from build123d import *

# Parameters (mm, degrees)
SKETCH1_R           = 12.5
BOSS_EXTRUDE2_DEPTH = 12
CUT_EXTRUDE3_REACH  = 14
SKETCH5_R           = 2.125
BOSS_EXTRUDE3_DEPTH = 12
SKETCH9_W           = 8
SKETCH9_H           = 10
CUT_EXTRUDE4_DEPTH  = 10
SKETCH10_W          = 8
SKETCH10_H          = 10
CUT_EXTRUDE5_DEPTH  = 10
SKETCH11_R          = 2
CUT_EXTRUDE6_DEPTH  = 21.229774891
SKETCH12_R          = 2
CUT_EXTRUDE7_DEPTH  = 30.012682497


with BuildPart() as part:
    # Sketch1 → Boss-Extrude2 (new body)
    with BuildSketch(Plane.XY):
        Circle(SKETCH1_R)
    extrude(amount=BOSS_EXTRUDE2_DEPTH)

    # Sketch5 → Cut-Extrude3 (cut, up to next)
    with BuildSketch(Plane.XY.offset(12), mode=Mode.PRIVATE) as cut_extrude3_sk1:
        Circle(SKETCH5_R)
    cut_extrude3_tool1 = extrude(cut_extrude3_sk1.sketch, amount=-CUT_EXTRUDE3_REACH, mode=Mode.PRIVATE) & part.part
    add(cut_extrude3_tool1.solids().sort_by_distance((0, 0, 12))[0], mode=Mode.SUBTRACT)

    # Sketch6 → Boss-Extrude3 (add)
    with BuildSketch(Plane.XY):
        with BuildLine():
            Line((10.356157589, 7), (20.356157589, 7))
            Line((20.356157589, 7), (20.356157589, -7))
            Line((20.356157589, -7), (10.356157589, -7))
            ThreePointArc((10.356157589, -7), (12.5, 0), (10.356157589, 7))
        make_face()
        with BuildLine():
            Line((-24.231440373, -0.295461436), (-11.458506302, 4.995261088))
            ThreePointArc((-11.458506302, 4.995261088), (-12.259311424, -2.441164357), (-8.670952565, -9.003587153))
            Line((-8.670952565, -9.003587153), (-18.87387232, -13.229774891))
            Line((-18.87387232, -13.229774891), (-20.787289482, -8.610377228))
            Line((-20.787289482, -8.610377228), (-24.231440373, -0.295461436))
        make_face()
    extrude(amount=BOSS_EXTRUDE3_DEPTH)

    # Sketch9 → Cut-Extrude4 (cut)
    with BuildSketch(Plane(origin=(20.356157589, 0, 0), x_dir=(0, 0, -1), z_dir=(1, 0, 0))):
        with Locations((-6, 0)):
            Rectangle(SKETCH9_W, SKETCH9_H)
    extrude(amount=-CUT_EXTRUDE4_DEPTH, mode=Mode.SUBTRACT)

    # Sketch10 → Cut-Extrude5 (cut)
    with BuildSketch(Plane(origin=(-20.787289482, -8.610377228, 0), x_dir=(0, 0, 1), z_dir=(-0.923879533, -0.382683432, 0))):
        with Locations((6, 2)):
            Rectangle(SKETCH10_W, SKETCH10_H)
    extrude(amount=-CUT_EXTRUDE5_DEPTH, mode=Mode.SUBTRACT)

    # Sketch11 → Cut-Extrude6 (cut, through all)
    with BuildSketch(Plane(origin=(0, 7, 0), x_dir=(1, 0, 0), z_dir=(0, 1, 0))):
        with Locations((15.356157589, -6)):
            Circle(SKETCH11_R)
    extrude(amount=-CUT_EXTRUDE6_DEPTH, mode=Mode.SUBTRACT)

    # Sketch12 → Cut-Extrude7 (cut, through all)
    with BuildSketch(Plane(origin=(-3.444150891, 8.314915793, 0), x_dir=(0.923879533, 0.382683432, 0), z_dir=(-0.382683432, 0.923879533, 0))):
        with Locations((-15.587337893, -6)):
            Circle(SKETCH12_R)
    extrude(amount=-CUT_EXTRUDE7_DEPTH, mode=Mode.SUBTRACT)


solid = part.part
Verification items for the finished model (mm, model axes). A direction names the side the tool comes from. Coordinates: 2 decimals unless noted, no trailing zeros. Write each loop counter-clockwise with the first axis right and the second up, starting at its lowest first coordinate (ties: lowest second). Pieces come first, ordered by that corner, then holes. Notation, with made-up numbers: (48.25, 43.5) - (107.25, 43.5) arc R31 cw to (107.25, 76.5) - close; hole circle Ø10 at (-12.75, 44). An arc over 180 degrees is marked (long way). Answer as a JSON object with one key per item and string values.
(1) Gauge pin test, flat ends, axial feed: pin 1 Ø3 at (x, z) = (13.5, 3.5) entering from -Y; pin 2 Ø3 at (x, z) = (14.5, 7.5) entering from +Y; pin 3 Ø2.5 at (x, z) = (15.36, 6) entering from -Y; pin 4 Ø4 at (y, z) = (-8.5, 2.5) entering from -X. Record the tip position at first contact, or that the pin passes through.
Report:
{"pin 1": "y = -7", "pin 2": "y = 7", "pin 3": "through", "pin 4": "x = -21.64"}
(2) Tool access check on faces 1 (the cylindrical face through (-0.958, 12.463, 5.916)), 2 (the flat face through (15, 0, 10)), 3 (the flat face through (-12.34, -2.87, 5.94)). Record the directions out of +Z, -Z, +X, -X, +Y, -Y that give a thin tool (end or side, any length) a straight path to the whole face; none if there is none.
Report:
{"face 1": "+Z, -Z, +Y", "face 2": "+X", "face 3": "none"}
(3) Cross-section at D-D on y = 5.75. Record the cut outline in (x, z), plus the area to 3 significant figures.
Report:
{"outline": "(-11.1, 0) - (20.36, 0) - (20.36, 12) - (-11.1, 12) - close; hole circle Ø4 at (15.36, 6)", "area": "365 mm^2"}
(4) Cross-section at C-C on z = 6. Give the number of separate pieces and of enclosed holes in the cut face, plus the area to 3 significant figures.
Report:
{"separate pieces": "5", "enclosed holes": "1", "area": "517 mm^2"}
(5) Cross-section at B-B on x = 0. Record the cut outline in (y, z) (3 decimals).
Report:
{"outline": "(-12.5, 0) - (-2.125, 0) - (-2.125, 12) - (-12.5, 12) - close; (2.125, 0) - (12.5, 0) - (12.5, 12) - (2.125, 12) - close"}
(6) Thickness scan on line 1 along X through (y, z) = (-0.5, 8.5); line 2 along Y through (x, z) = (10.5, 4.75); line 3 along X through (y, z) = (-1.75, 2.5). Record the ranges inside material, lowest first.
Report:
{"line 1": "-24.15 to -19.5, -13.32 to -2.07, 2.07 to 10.36", "line 2": "-7 to -5, 5 to 7", "line 3": "-23.63 to -22.52, -12.81 to -1.21, 1.21 to 10.36"}
(7) Mould release check, pull along X, two halves, no side actions. Record for faces 4 (the flat face through (-19.354, 1.725, 4.583)), 5 (the flat face through (-14.835, -11.557, 5.916)), 6 (the flat face through (18, -7, 6)): pulls with the +X half, pulls with the -X half, needs draft (parallel to the pull), parting line crosses it, or undercut.
Report:
{"face 4": "pulls with the -X half", "face 5": "undercut", "face 6": "needs draft"}
